```python
from build123d import *

# Parameters (mm, degrees)
F2_R     = 2
F3_DEPTH = 2.5
F4_R     = 2
F5_DEPTH = 3
F6_R     = 1
F7_DEPTH = 2


with BuildPart() as f1:
    # F0 (on Right) → F1 (revolve)
    with BuildSketch(Plane.YZ):
        with BuildLine():
            ThreePointArc((0, -2.5), (2.5, 0), (0, 2.5))
            Line((0, 2.5), (0, 2))
            ThreePointArc((0, 2), (2, 0), (0, -2))
            Line((0, -2), (0, -2.5))
        make_face()
    revolve(axis=Axis((0, 0, 0), (0, 0, -1)))

    # F2 (on Right) → F3 (cut)
    with BuildSketch(Plane.YZ):
        Circle(F2_R)
    extrude(amount=-F3_DEPTH, mode=Mode.SUBTRACT)

    # F4 (on Right) → F5 (join)
    with BuildSketch(Plane.YZ):
        Circle(F4_R)
    extrude(amount=F5_DEPTH)

    # F6 (on face) → F7 (join)
    with BuildSketch(Plane.YZ.offset(3)):
        with BuildLine():
            ThreePointArc((-2, 0), (0, -2), (2, 0))
            ThreePointArc((2, 0), (0, 2), (-2, 0))
        make_face()
        with BuildLine():
            ThreePointArc((-2, 0), (0, 2), (2, 0))
            Line((2, 0), (2, 15))
            ThreePointArc((2, 15), (0, 13), (-2, 15))
            Line((-2, 15), (-2, 0))
        make_face()
        with BuildLine():
            ThreePointArc((-2, 15), (0, 13), (2, 15))
            ThreePointArc((2, 15), (0, 17), (-2, 15))
        make_face()
        with Locations((0, 15)):
            Circle(F6_R, mode=Mode.SUBTRACT)
    extrude(amount=F7_DEPTH)

    # F8 (on face) → F9 (revolve, cut)
    with BuildSketch(Plane(origin=(0, 0, 0), x_dir=(0, -1, 0), z_dir=(-1, 0, 0))):
        with BuildLine():
            Line((0, 2), (0, -2))
            ThreePointArc((0, -2), (1.4142135624, -1.4142135624), (2, 0))
            ThreePointArc((2, 0), (1.4142135624, 1.4142135624), (0, 2))
        make_face()
    revolve(axis=Axis((0, 0, 0), (0, 0, 1)), mode=Mode.SUBTRACT)


solid = f1.part
```
Here's how the part is built. I have some questions about the finished solid (model axes, mm). Round coordinates to 2 decimals unless told otherwise and drop trailing zeros. Order: outer loops, then holes, each group sorted by start corner. A loop starts at its lowest first (then second) coordinate and runs counter-clockwise, first axis right, second up. Notation, with made-up numbers: M 25.5,-0.75 L 48.5,-0.75 A27 ccw 48.5,18.25 Z; hole C -29,13 d11. An arc over 180 degrees is marked long. Answer in a Markdown table with one row per item.
Item 1: I'm going to push flat-ended pins straight in: pin 1 (3 mm diameter, centred on y = -0.5, z = 7.5, fed in from -X); pin 2 (1.6 mm diameter, centred on y = 0, z = 15, fed in from +X); pin 3 (0.6 mm diameter, centred on x = 4.5, z = 9.5, fed in from -Y); pin 4 (2 mm diameter, centred on x = 4, z = 15, fed in from +Y). Where does each tip first touch, or does it pass through?
A:
| item | result |
|---|---|
| pin 1 | stops at x = 3 |
| pin 2 | passes through |
| pin 3 | stops at y = -2 |
| pin 4 | stops at y = 2 |
Item 2: Imagine slicing it at A-A, the plane y = 0. Write out the boundary of the cut face in (x, z).
A:
| item | result |
|---|---|
| outline | M -1.5,-2 A2.5 ccw 1.5,-2 L 5,-2 L 5,14 L 3,14 L 3,2 L 1.5,2 A2.5 ccw -1.5,2 L 0,2 A2 cw 0,-2 Z; M 3,16 L 5,16 L 5,17 L 3,17 Z |
Item 3: Imagine slicing it at C-C, the plane y = -1.3. Write out the boundary of the cut face in (x, z).
A:
| item | result |
|---|---|
| outline | M -1.5,-1.52 A2.14 ccw 1.5,-1.52 L 5,-1.52 L 5,16.52 L 3,16.52 L 3,1.52 L 1.5,1.52 A2.14 ccw -1.5,1.52 L 0,1.52 A1.52 cw 0,-1.52 Z |
Item 4: Imagine slicing it at D-D, the plane z = 12.5. Write out the boundary of the cut face in (x, y).
A:
| item | result |
|---|---|
| outline | M 3,-2 L 5,-2 L 5,2 L 3,2 Z |
Item 5: Imagine slicing it at B-B, the plane x = 4.5. Write out the boundary of the cut face in (y, z).
A:
| item | result |
|---|---|
| outline | M -2,0 A2 ccw 2,0 L 2,15 A2 ccw -2,15 Z; hole C 0,15 d2 |
Item 6: Thinking about a two-plate mould opening in Y: for faces 1 (the face through (3, 0, 9)), 2 (the face through (-1, 0, -2)), 3 (the face through (4, 0, 14)), 4 (the face through (3, 0, -2)), which applies, +Y half, -Y half, draft (parallel to the pull), parting line (faces both ways), or undercut?
A:
| item | result |
|---|---|
| face 1 | draft |
| face 2 | undercut |
| face 3 | undercut |
| face 4 | parting line |
Item 7: If I drill on L1, parallel to Z at x = 4.1, y = 0; L2, parallel to X at y = -0.1, z = 5; L3, parallel to Z at x = -0.5, y = 0, over which ranges is the centre line in solid material (lowest first)? Write a range as from..to.
A:
| item | result |
|---|---|
| L1 | z = -2..14, 16..17 |
| L2 | x = 3..5 |
| L3 | z = -2.45..-2, 2..2.45 |
